from build123d import *

# Parameters (mm, degrees)
SKETCH023_R  = 1.7
PAD012_DEPTH = 3
PAD013_DEPTH = 5


with BuildPart() as part:
    # Sketch023 → Pad012 (new body)
    with BuildSketch(Plane(origin=(0, 75, 0), x_dir=(-1, 0, 0), z_dir=(0, 1, 0))):
        Polygon((-15.7, -7.5), (-15.7, 9.4), (-12, 9.4), (-8.3, 9.4), (-8.3, -7.5), align=None)
        with Locations((-12, 4)):
            Circle(SKETCH023_R, mode=Mode.SUBTRACT)
    pad012 = extrude(amount=PAD012_DEPTH)

    # Sketch025 (on Face5 of Pad012) → Pad013 (join)
    with BuildSketch(Plane(origin=(0, 0, -7.5), x_dir=(1, 0, 0), z_dir=(0, 0, -1))):
        with BuildLine():
            ThreePointArc((0, -77.043425), (34.5032756474, -63.2307704346), (49.943278179, -29.4243837841))
            ThreePointArc((54.9376070845, -29.6624568488), (52.5594789409, -27.0462605473), (49.943278179, -29.4243837841))
            ThreePointArc((0, -82.043425), (37.9536114771, -66.8494970976), (54.9376070845, -29.6624568488))
            Line((0, -77.043425), (0, -82.043425))
        make_face()
    pad013 = extrude(amount=PAD013_DEPTH)

    # Mirrored007: Pad013, Pad012 across Sketch025 V_Axis
    add(pad013.mirror(Plane(origin=(0, 0, -7.5), x_dir=(0, 0, -1), z_dir=(1, 0, 0))))
    add(pad012.mirror(Plane(origin=(0, 0, -7.5), x_dir=(0, 0, -1), z_dir=(1, 0, 0))))


solid = part.part
Check sheet for the modelled part. Datum: model origin and axes. Units: mm. A direction names the side the tool comes from. Round coordinates to 2 decimals unless told otherwise and drop trailing zeros. Order: outer loops, then holes, each group sorted by start corner. A loop starts at its lowest first (then second) coordinate and runs counter-clockwise, first axis right, second up.
(1) Scan lines: probe 1 along Z at (x, y) = (-12, 75.65); probe 2 along X at (y, z) = (77, 6.25); probe 3 along Y at (x, z) = (10.5, -7). Record each from-to range of solid material in increasing order.
(2) Draft check along X on faces 1 (the flat face through (12, 76, 9.4)), 2 (the cylindrical face through (-10.43, 76.48, 3.35)), 3 (the flat face through (-15.7, 76, 1)). Enter one of: pulls with the +X half, pulls with the -X half, needs draft (parallel to the pull), parting line crosses it, or undercut.
(3) Access from +Z, -Z, +X, -X, +Y, -Y to the whole of each face (thin tool, end or side, straight path). Record for faces 4 (the flat face through (12, 78, 1)), 5 (the flat face through (8.3, 76, 1)), 6 (the flat face through (-12, 75, 1)).
(4) Cross-section at C-C, the plane z = 4. Enter the section's corners in (x, y).
(5) Go/stop test with flat-tipped pins: P1, Ø3.5, axis at y = 77, z = -2, coming from the -X side; P2, Ø0.9, axis at y = 76.5, z = -3, coming from the +X side; P3, Ø3.5, axis at x = 11.5, z = 0.5, coming from the +Y side; P4, Ø2.5, axis at x = 12, z = 4, coming from the -Y side. Record where each tip stops, or that it passes through.
(6) Cross-section at B-B, the plane y = 65.5. Enter the section's corners in (x, z).
(7) Cross-section at A-A, the plane z = -1.75. Enter the section's corners in (x, y), and give its area (3 significant figures).
(8) Cross-section at D-D, the plane x = -12. Enter the section's corners in (y, z).
Check sheet entries:
1. probe 1: z = -12.5 to 2.3, 5.7 to 9.4
1. probe 2: x = -15.7 to -8.3, 8.3 to 15.7
1. probe 3: y = 75 to 78
2. face 1: needs draft
2. face 2: undercut
2. face 3: pulls with the -X half
3. face 4: +Z, +X, -X, +Y
3. face 5: +Z, +Y, -Y
3. face 6: +Z, +X, -X, -Y
4. outline: (-15.7, 75) - (-13.7, 75) - (-13.7, 78) - (-15.7, 78) - close; (-10.3, 75) - (-8.3, 75) - (-8.3, 78) - (-10.3, 78) - close; (8.3, 75) - (10.3, 75) - (10.3, 78) - (8.3, 78) - close; (13.7, 75) - (15.7, 75) - (15.7, 78) - (13.7, 78) - close
5. P1: stops at x = -15.7
5. P2: stops at x = 15.7
5. P3: stops at y = 78
5. P4: passes through
6. outline: (-39.32, -12.5) - (-31.95, -12.5) - (-31.95, -7.5) - (-39.32, -7.5) - close; (31.95, -12.5) - (39.32, -12.5) - (39.32, -7.5) - (31.95, -7.5) - close
7. outline: (-15.7, 75) - (-8.3, 75) - (-8.3, 78) - (-15.7, 78) - close; (8.3, 75) - (15.7, 75) - (15.7, 78) - (8.3, 78) - close
7. area: 44.4 mm2
8. outline: (75, -7.5) - (75.58, -7.5) - (75.58, -12.5) - (80.72, -12.5) - (80.72, -7.5) - (78, -7.5) - (78, 2.3) - (75, 2.3) - close; (75, 5.7) - (78, 5.7) - (78, 9.4) - (75, 9.4) - close
